Here's how the part is built. I have some questions about the finished solid (model axes, mm). A direction names the side the tool comes from. Give positions to 0.01 mm unless a question says otherwise; leave off trailing zeros. Loops run counter-clockwise (first coordinate to the right, second up) from the corner with the lowest first, then second, coordinate; pieces in that order, holes last. Notation, with made-up numbers: M 28.5,51.5 L 33.5,51.5 A13 cw 33.5,74.5 Z; hole C 52.25,15.25 d9. An arc over 180 degrees is marked long. Write item = value, one per line. Start each with the question number.
```python
from build123d import *

# Parameters (mm, degrees)
F0_R          = 24.511
F0_R_2        = 16.8275
F0_R_3        = 12.7
F1_DEPTH      = 18.0975
F2_DEPTH      = 29.0322
F2_DEPTH_BACK = 5.08
F3_DEPTH      = 29.0332


with BuildPart() as f1:
    # F0 (on Top) → F1 (new body)
    with BuildSketch(Plane.XY):
        Circle(F0_R)
        Circle(F0_R_2, mode=Mode.SUBTRACT)
        Circle(F0_R_2)
        Circle(F0_R_3, mode=Mode.SUBTRACT)
        Circle(F0_R_3)
    extrude(amount=F1_DEPTH)

    # F0 (on Top) → F2 (join, two sides)
    with BuildSketch(Plane.XY) as f2_sk:
        Circle(F0_R_2)
        Circle(F0_R_3, mode=Mode.SUBTRACT)
    extrude(amount=F2_DEPTH)
    extrude(f2_sk.sketch, amount=-F2_DEPTH_BACK)

    # F3 (cut, through all): a face of the model
    f3_faces = [f1.faces().sort_by_distance(p)[0] for p in [
        (0, 0, 0),
    ]]
    extrude(f3_faces, amount=-F3_DEPTH, mode=Mode.SUBTRACT)


solid = f1.part
```
Q1. We'd pull the mould along X, two halves only. Please class faces 1 (the cylindrical face through (-19.451, -14.915, 8.922)), 2 (the cylindrical face through (-2.75, -12.4, 12.21)), 3 (the flat face through (2, 13, 29.032)): pulls with the +X half, pulls with the -X half, needs draft (parallel to the pull), parting line crosses it, or undercut.
Q2. If we section it at D-D, the plane x = 13.5: List the corners of the cut face in (y, z) for me, then the cut area to 3 significant figures.
Q3. Will these pins go through, and if not, where does the flat tip stop? pin 1 (20.5 mm diameter, centred on x = 0, y = 0, fed in from +Z); pin 2 (10 mm diameter, centred on x = -12.5, z = 6.5, fed in from +Y); pin 3 (12 mm diameter, centred on y = 12.5, z = 6.5, fed in from +X); pin 4 (1.5 mm diameter, centred on y = -19, z = 2, fed in from +X).
Q4. On a 3-axis mill with a long thin cutter (end or side, diameter ignored), from which of +Z, -Z, +X, -X, +Y, -Y can I reach the whole of each face in a straight line? I mean faces 4 (the flat face through (2, 13, -5.08)), 5 (the flat face through (-6, -16, 18.098)), 6 (the cylindrical face through (-3.648, -16.427, -2.504)). Say none if no direction works.
Q5. If we section it at C-C, the plane z = 6: List the corners of the cut face in (x, y) for me, then the cut area to 3 significant figures.
Q6. If we section it at A-A, the plane x = 0: List the corners of the cut face in (y, z) for me.
Q7. If I drill on line 1 along Y through (x, z) = (0, 12); line 2 along Y through (x, z) = (0, 20); line 3 along X through (y, z) = (5.5, 23.5), over which ranges is the centre line in solid material (lowest first)?
Resolved:
q1.face_1 = parting line crosses it
q1.face_2 = undercut
q1.face_3 = needs draft
q2.outline = M -20.46,0 L -10.05,0 L -10.05,-5.08 L 10.05,-5.08 L 10.05,0 L 20.46,0 L 20.46,18.1 L 10.05,18.1 L 10.05,29.03 L -10.05,29.03 L -10.05,18.1 L -20.46,18.1 Z
q2.area = 1,060 mm²
q3.pin_1 = through
q3.pin_2 = 23.34
q3.pin_3 = 23.63
q3.pin_4 = 16.36
q4.face_4 = -Z, +X, -X, +Y, -Y
q4.face_5 = +Z
q4.face_6 = -Z
q5.outline = C 0,0 d49.02; hole C 0,0 d25.4
q5.area = 1,380 mm²
q6.outline = M -24.51,0 L -16.83,0 L -16.83,-5.08 L -12.7,-5.08 L -12.7,29.03 L -16.83,29.03 L -16.83,18.1 L -24.51,18.1 Z; M 12.7,-5.08 L 16.83,-5.08 L 16.83,0 L 24.51,0 L 24.51,18.1 L 16.83,18.1 L 16.83,29.03 L 12.7,29.03 Z
q7.line_1 = -24.51 to -12.7, 12.7 to 24.51
q7.line_2 = -16.83 to -12.7, 12.7 to 16.83
q7.line_3 = -15.9 to -11.45, 11.45 to 15.9
